Verification items for this drawing (mm, ordinates from the low corner). A direction names the side the tool comes from. Coordinates: 2 decimals unless noted, no trailing zeros. Loops run counter-clockwise (first coordinate to the right, second up) from the corner with the lowest first, then second, coordinate; pieces in that order, holes last. Notation, with made-up numbers: M 83.25,41.25 L 120.25,41.25 A6 cw 120.25,52.25 Z; hole C -11.75,-38.5 d6. An arc over 180 degrees is marked long. Write each question's results on one line, items separated by ' | '. Start each with the question number.
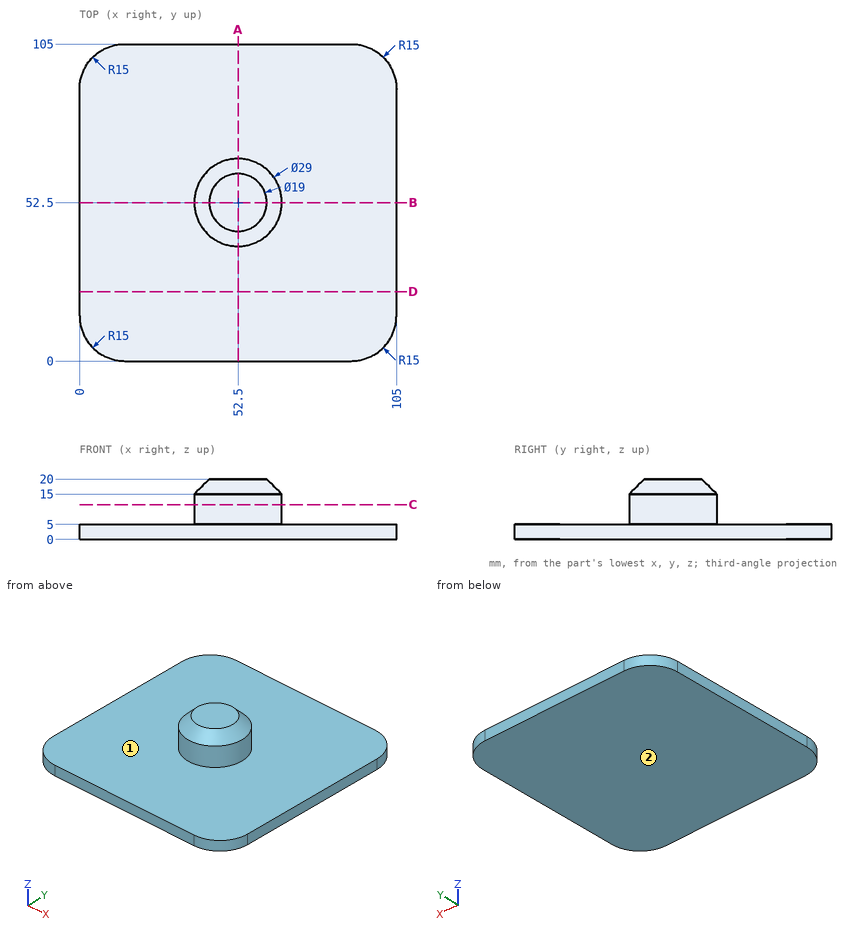
Item 1: Tool access check on the marked faces 1 and 2. Record the directions out of +Z, -Z, +X, -X, +Y, -Y that give a thin tool (end or side, any length) a straight path to the whole face; none if there is none.
Item 2: Thickness scan on line 1 (Z direction, x = 7, y = 34); line 2 (X direction, y = 60.5, z = 11.75); line 3 (X direction, y = 47, z = 9.5). Record the ranges inside material, lowest first.
Item 3: Section check C-C (z = 11.5). Record the cut outline in (x, y), plus the area to 3 significant figures.
Item 4: Section check A-A (x = 52.5). Record the cut outline in (y, z), plus the area to 3 significant figures.
Item 5: Depth check by flat-ended pin: P1, Ø6, axis at y = 54.5, z = 13, coming from the +X side; P2, Ø10, axis at x = 88, y = 12.5, coming from the +Z side; P3, Ø12, axis at y = 37, z = 13, coming from the +X side. Enter the tip coordinate at first touch or a pass-through.
Item 6: Section check D-D (y = 23). Record the cut outline in (x, z), plus the area to 3 significant figures.
Computed values:
1) face 1: +Z | face 2: -Z, +X, -X, +Y, -Y
2) line 1: z = 0 to 5 | line 2: x = 40.41 to 64.59 | line 3: x = 39.08 to 65.92
3) outline: C 52.5,52.5 d29 | area: 661 mm²
4) outline: M 0,0 L 105,0 L 105,5 L 67,5 L 67,15 L 62,20 L 43,20 L 38,15 L 38,5 L 0,5 Z | area: 935 mm²
5) P1: stops at x = 67 | P2: stops at z = 5 | P3: stops at x = 63.45
6) outline: M 0,0 L 105,0 L 105,5 L 0,5 Z | area: 525 mm²
